Autodesk Inventor part; units mm, degrees
ref_plane "YZ Plane" through (0, 0, 0) normal (1, 0, 0) x (0, 1, 0)
ref_plane "XZ Plane" through (0, 0, 0) normal (0, 1, 0) x (-1, 0, 0)
ref_plane "XY Plane" through (0, 0, 0) normal (0, 0, 1) x (1, 0, 0)
sketch "Skizze1" plane through (0, 0, 0) normal (0, 0, 1) x (1, 0, 0)
  line L0 (-3, 1.5) -> (5, 1.5)
  line L1 (-3, 1.5) -> (-3, 3.5)
  line L2 (-3, 3.5) -> (6, 3.5)
  line L3 (6, 3.5) -> (9, 2.5)
  line L4 (9, 2.5) -> (9, 0)
  line L5 (5, -1.5) -> (-3, -1.5)
  line L6 (-3, -1.5) -> (-3, -3.5)
  line L7 (-3, -3.5) -> (6, -3.5)
  line L8 (6, -3.5) -> (9, -2.5)
  line L9 (9, -2.5) -> (9, 0)
  line L10 (5, -1.5) -> (5, 1.5)
  point P0 (0, 0)
  point P1 (5, 0)
  dimension "d0" = 3
  dimension "d1" = 2
  dimension "d2" = 3
  dimension "d4" = 5
  dimension "d5" = 4
  dimension "d6" = 1
  dimension "d7" = 3
extrude "Extrusion1" add sketch "Skizze1" along normal mid plane 5
sketch "Skizze2" plane through (-3, 3.5, 2.5) normal (0, 1, 0) x (1, 0, 0)
  line L0 (3, 6) -> (3, -1)
  line L1 (14.4, 2.5) -> (-2.4, 2.5)
  circle A0 centre (3, 2.5) radius 1
  dimension "d10" = 2
extrude "Extrusion2" cut sketch "Skizze2" along normal through all both and the other way through all
sketch "Skizze3" plane through (9, -2.5, 2.5) normal (1, 0, 0) x (0, 0, -1)
  circle A0 centre (2.5, 2.5) radius 2.5
  line L0 (5, 5) -> (5, 0)
extrude "Extrusion3" add sketch "Skizze3" along normal blind 2
properties part number "Schakel"
CAD build for the part. Positions are in the model's coordinates, mm. A direction names the side the tool comes from. Give positions to 0.01 mm unless a question says otherwise; leave off trailing zeros. Order: outer loops, then holes, each group sorted by start corner. A loop starts at its lowest first (then second) coordinate and runs counter-clockwise, first axis right, second up. Notation, with made-up numbers: (32, 30.25) - (78, 30.25) arc R36 cw to (78, 66.25) - close; hole circle Ø5 at (-33.75, 27). An arc over 180 degrees is marked (long way). Answer in a Markdown table with one row per item.
1. Probe probe 1 along Y at (x, z) = (-1, -1.5); probe 2 along Z at (x, y) = (0, -3.1); probe 3 along X at (y, z) = (0.5, -0.9). List the from-to ranges inside material, lowest first. Write a range as [from, to].
Data:
| item | result |
|---|---|
| probe 1 | y = [-3.5, -1.5], [1.5, 3.5] |
| probe 2 | z = [-2.5, -1], [1, 2.5] |
| probe 3 | x = [5, 11] |
2. Saw through at A-A, the plane x = 4.5. Give the cut face in (y, z).
Data:
| item | result |
|---|---|
| outline | (-3.5, -2.5) - (-1.5, -2.5) - (-1.5, 2.5) - (-3.5, 2.5) - close; (1.5, -2.5) - (3.5, -2.5) - (3.5, 2.5) - (1.5, 2.5) - close |
3. Tool access for faces 1 (the flat face through (9, 2, 2)), 2 (the cylindrical face through (9.99, 2.44, 0.54)), 3 (the flat face through (9, -2, -2)), 4 (the flat face through (9, 2, -2)): list every direction of +Z, -Z, +X, -X, +Y, -Y with a clear straight run to the whole face (end or side of a thin tool).
Data:
| item | result |
|---|---|
| face 1 | +Z, +X, +Y |
| face 2 | +X |
| face 3 | -Z, +X, -Y |
| face 4 | -Z, +X, +Y |
4. Pull direction Y, two halves, no side cores. Call faces 5 (the flat face through (7.5, 3, 0)), 6 (the flat face through (1, 1.5, -1)), 7 (the flat face through (11, 0, 0)), 8 (the flat face through (5, 0, 0)): pulls with the +Y half, pulls with the -Y half, needs draft (parallel to the pull), parting line crosses it, or undercut.
Data:
| item | result |
|---|---|
| face 5 | pulls with the +Y half |
| face 6 | undercut |
| face 7 | needs draft |
| face 8 | undercut |
5. Saw through at D-D, the plane z = -0.3. Count the separate pieces of the cut face and the enclosed holes in it, plus the area to 3 significant figures.
Data:
| item | result |
|---|---|
| separate pieces | 3 |
| enclosed holes | 0 |
| area | 59.3 mm² |
6. Saw through at B-B, the plane y = 2. Give the cut face in (x, z), plus the area to 3 significant figures.
Data:
| item | result |
|---|---|
| outline | (-3, -2.5) - (9, -2.5) - (9, -1.5) - (11, -1.5) - (11, 1.5) - (9, 1.5) - (9, 2.5) - (-3, 2.5) - close; hole circle Ø2 at (0, 0) |
| area | 62.9 mm² |
7. Saw through at C-C, the plane x = 0. Give the cut face in (y, z), plus the area to 3 significant figures.
Data:
| item | result |
|---|---|
| outline | (-3.5, -2.5) - (-1.5, -2.5) - (-1.5, -1) - (-3.5, -1) - close; (-3.5, 1) - (-1.5, 1) - (-1.5, 2.5) - (-3.5, 2.5) - close; (1.5, -2.5) - (3.5, -2.5) - (3.5, -1) - (1.5, -1) - close; (1.5, 1) - (3.5, 1) - (3.5, 2.5) - (1.5, 2.5) - close |
| area | 12.0 mm² |
